from build123d import *

# Parameters (mm, degrees)
SKETCH5_W           = 25.4
SKETCH5_H           = 25.4
BOSS_EXTRUDE2_DEPTH = 2.54
SKETCH6_W           = 25.4
SKETCH6_H           = 3.086684186
BOSS_EXTRUDE3_DEPTH = 49.9364
SKETCH7_R           = 1.27
CUT_EXTRUDE1_DEPTH  = 49.9364
SKETCH8_R           = 1.503583718
CUT_EXTRUDE2_DEPTH  = 49.9364
SKETCH9_W           = 11.960422389
SKETCH9_H           = 7.288882616
SKETCH9_W_2         = 11.577688012
SKETCH9_H_2         = 7.115600704
CUT_EXTRUDE4_DEPTH  = 5.08
SKETCH10_W          = 13.617142972
SKETCH10_H          = 13.156114308
SKETCH10_H_2        = 13.156114309
CUT_EXTRUDE5_DEPTH  = 2.032
SKETCH12_W          = 25.4
SKETCH12_H          = 5.336540019
CUT_EXTRUDE6_DEPTH  = 2.54


with BuildPart() as part:
    # Sketch5 → Boss-Extrude2 (new body)
    with BuildSketch(Plane(origin=(0, 0, 0), x_dir=(0, 0, -1), z_dir=(1, 0, 0))):
        with Locations((6.544263828, 0.143373815)):
            Rectangle(SKETCH5_W, SKETCH5_H)
    extrude(amount=-BOSS_EXTRUDE2_DEPTH)

    # Sketch6 → Boss-Extrude3 (add)
    with BuildSketch(Plane(origin=(0, 0, 0), x_dir=(0, 0, -1), z_dir=(1, 0, 0))):
        with Locations((6.544263828, -11.013284092)):
            Rectangle(SKETCH6_W, SKETCH6_H)
    extrude(amount=BOSS_EXTRUDE3_DEPTH)

    # Sketch7 → Cut-Extrude1 (cut)
    with BuildSketch(Plane(origin=(0, -9.469941999, 0), x_dir=(1, 0, 0), z_dir=(0, 1, 0))):
        with Locations(Location((2.479766783, 16.6315447, 0), (0, 0, 270))):
            Circle(SKETCH7_R)
        with Locations(Location((47.725207241, -3.210779596, 0), (0, 0, 270))):
            Circle(SKETCH7_R)
        with Locations(Location((47.723516777, 16.630771834, 0), (0, 0, 270))):
            Circle(SKETCH7_R)
        with Locations(Location((2.481517748, -3.212205223, 0), (0, 0, 270))):
            Circle(SKETCH7_R)
    extrude(amount=-CUT_EXTRUDE1_DEPTH, mode=Mode.SUBTRACT)

    # Sketch8 → Cut-Extrude2 (cut)
    with BuildSketch(Plane(origin=(0, 0, 0), x_dir=(0, 0, -1), z_dir=(1, 0, 0))):
        with Locations((6.760840433, 3.230058001)):
            Circle(SKETCH8_R)
    extrude(amount=-CUT_EXTRUDE2_DEPTH, mode=Mode.SUBTRACT)

    # Sketch9 → Cut-Extrude4 (cut)
    with BuildSketch(Plane(origin=(0, -9.469941999, 0), x_dir=(1, 0, 0), z_dir=(0, 1, 0))):
        with Locations((24.323492834, 15.59982252)):
            Rectangle(SKETCH9_W, SKETCH9_H)
        with Locations((24.247688593, -2.66541828)):
            Rectangle(SKETCH9_W_2, SKETCH9_H_2)
    extrude(amount=-CUT_EXTRUDE4_DEPTH, mode=Mode.SUBTRACT)

    # Sketch10 → Cut-Extrude5 (cut)
    with BuildSketch(Plane(origin=(0, -9.469941999, 0), x_dir=(1, 0, 0), z_dir=(0, 1, 0))):
        with Locations((6.733736813, 6.670159659)):
            Rectangle(SKETCH10_W, SKETCH10_H)
        with Locations((43.127828514, 6.607211743)):
            Rectangle(SKETCH10_W, SKETCH10_H_2)
    extrude(amount=-CUT_EXTRUDE5_DEPTH, mode=Mode.SUBTRACT)

    # Sketch12 → Cut-Extrude6 (cut)
    with BuildSketch(Plane(origin=(0, 0, 0), x_dir=(0, 0, -1), z_dir=(1, 0, 0))):
        with Locations((6.544263828, 10.175103806)):
            Rectangle(SKETCH12_W, SKETCH12_H)
    extrude(amount=-CUT_EXTRUDE6_DEPTH, mode=Mode.SUBTRACT)


solid = part.part
Input: part model. Units: mm. Frame: model coordinates. A direction names the side the tool comes from. Give positions to 0.01 mm unless a question says otherwise; leave off trailing zeros. Loops run counter-clockwise (first coordinate to the right, second up) from the corner with the lowest first, then second, coordinate; pieces in that order, holes last. Notation, with made-up numbers: M -5.5,-35 L 24.5,-35 A35 ccw 24.5,2 Z; hole C 84,-26.5 d9. An arc over 180 degrees is marked long. Use CSV: the item, a comma, the result in double quotes.
(1) Section D-D, the plane x = 3. Return loops of the section in (y, z).
Outcome:
outline,"M -12.56,-19.24 L -9.47,-19.24 L -9.47,-17.79 L -12.56,-17.79 Z; M -12.56,-15.47 L -9.47,-15.47 L -9.47,-13.25 L -11.5,-13.25 L -11.5,-0.09 L -9.47,-0.09 L -9.47,2.05 L -12.56,2.05 Z; M -12.56,4.37 L -9.47,4.37 L -9.47,6.16 L -12.56,6.16 Z"
(2) Section C-C, the plane z = 3. Return loops of the section in (x, y).
Outcome:
outline,"M -2.54,-12.56 L 1.23,-12.56 L 1.23,-9.47 L 0,-9.47 L 0,7.51 L -2.54,7.51 Z; M 3.73,-12.56 L 18.46,-12.56 L 18.46,-9.47 L 3.73,-9.47 Z; M 30.04,-12.56 L 46.47,-12.56 L 46.47,-9.47 L 30.04,-9.47 Z; M 48.98,-12.56 L 49.94,-12.56 L 49.94,-9.47 L 48.98,-9.47 Z"
(3) Pull-direction query (Z, two-part tool) for faces 1 (the face through (18.343, -11, -16)), 2 (the face through (40, -11, -19.244)), 3 (the face through (7, -10, -13.248)), 4 (the face through (-0.075, -10, -7)); classes: pulls with the +Z half, pulls with the -Z half, needs draft (parallel to the pull), parting line crosses it, or undercut.
Outcome:
face 1,"needs draft"
face 2,"pulls with the -Z half"
face 3,"undercut"
face 4,"undercut"
(4) Set-up query: faces 5 (the face through (13.542, -10, -7)), 6 (the face through (30, -9.47, -6)), 7 (the face through (-2.54, -2, -6)), 8 (the face through (43, -11.502, -7)), 9 (the face through (24, -11, -11.955)). Return all of +Z, -Z, +X, -X, +Y, -Y with unobstructed straight access to the full face (end or side cutting, diameter ignored); none if empty.
Outcome:
face 5,"+Y"
face 6,"+Z, -Z, +X, +Y"
face 7,"+Z, -Z, -X, +Y, -Y"
face 8,"+X, +Y"
face 9,"-Z, +Y, -Y"
(5) Section A-A, the plane x = 12.5. Return loops of the section in (y, z), plus the area to 3 significant figures.
Outcome:
outline,"M -12.56,-19.24 L -9.47,-19.24 L -9.47,-13.25 L -11.5,-13.25 L -11.5,-0.09 L -9.47,-0.09 L -9.47,6.16 L -12.56,6.16 Z"
area,"51.7 mm²"
(6) Material intervals for L1, parallel to X at y = -5, z = -2; L2, parallel to Y at x = 5.5, z = -3.25; L3, parallel to Y at x = 17.5, z = -0.75, sorted ascending. Write a range as [from, to].
Outcome:
L1,"x = [-2.54, 0]"
L2,"y = [-12.56, -11.5]"
L3,"y = [-12.56, -9.47]"
(7) Pin query (flat end, axial travel): P1, Ø8.5, axis at y = -2.5, z = -8.5, coming from the +X side; P2, Ø6.5, axis at x = 3.5, z = -5.5, coming from the +Y side; P3, Ø2, axis at x = 2.48, z = -16.63, coming from the +Y side; P4, Ø1.5, axis at x = 21.5, y = -11.5, coming from the -Z side. Return the tip coordinate at first contact, or that it passes through.
Outcome:
P1,"stops at x = 0"
P2,"stops at y = -11.5"
P3,"passes through"
P4,"stops at z = -11.96"
(8) Section B-B, the plane z = -11. Return loops of the section in (x, y).
Outcome:
outline,"M -2.54,-12.56 L 49.94,-12.56 L 49.94,-11.5 L 36.32,-11.5 L 36.32,-9.47 L 13.54,-9.47 L 13.54,-11.5 L -0.07,-11.5 L -0.07,-9.47 L 0,-9.47 L 0,7.51 L -2.54,7.51 Z"
